Input: part model. Units: mm. Frame: model coordinates. Face numbers are marked on the shaded views. A direction names the side the tool comes from. Coordinates: 2 decimals unless noted, no trailing zeros. Loops run counter-clockwise (first coordinate to the right, second up) from the corner with the lowest first, then second, coordinate; pieces in that order, holes last.
```python
from build123d import *

# Parameters (mm, degrees)
SKETCH1_W           = 24.634
SKETCH1_H           = 13
BOSS_EXTRUDE1_DEPTH = 10
SKETCH4_W           = 70
SKETCH4_H           = 13
BOSS_EXTRUDE4_DEPTH = 15
FILLET2_R           = 5
SKETCH11_R          = 2.68
CUT_EXTRUDE3_DEPTH  = 26
SKETCH12_R          = 4.61
CUT_EXTRUDE4_DEPTH  = 6


with BuildPart() as part:
    # Sketch1 → Boss-Extrude1 (new body)
    with BuildSketch(Plane.XY):
        with Locations((12.317, 6.5)):
            Rectangle(SKETCH1_W, SKETCH1_H)
    extrude(amount=BOSS_EXTRUDE1_DEPTH)

    # Sketch4 → Boss-Extrude4 (add)
    with BuildSketch(Plane.XY.offset(10)):
        with Locations((35, 6.5)):
            Rectangle(SKETCH4_W, SKETCH4_H)
    extrude(amount=BOSS_EXTRUDE4_DEPTH)

    # Fillet2
    fillet2_edges = [part.edges().sort_by_distance(p)[0] for p in [
        (24.634, 6.5, 10),
    ]]
    fillet(fillet2_edges, radius=FILLET2_R)

    # Sketch11 → Cut-Extrude3 (cut, through all)
    with BuildSketch(Plane(origin=(0, 0, 0), x_dir=(-1, 0, 0), z_dir=(0, 0, -1))):
        with Locations((-5.067, 6.5)):
            Circle(SKETCH11_R)
        with Locations((-19.567, 6.5)):
            Circle(SKETCH11_R)
    extrude(amount=-CUT_EXTRUDE3_DEPTH, mode=Mode.SUBTRACT)

    # Sketch12 → Cut-Extrude4 (cut)
    with BuildSketch(Plane.XY.offset(25)):
        with Locations((5.067, 6.5)):
            Circle(SKETCH12_R)
        with Locations((19.567, 6.5)):
            Circle(SKETCH12_R)
    extrude(amount=-CUT_EXTRUDE4_DEPTH, mode=Mode.SUBTRACT)


solid = part.part
```
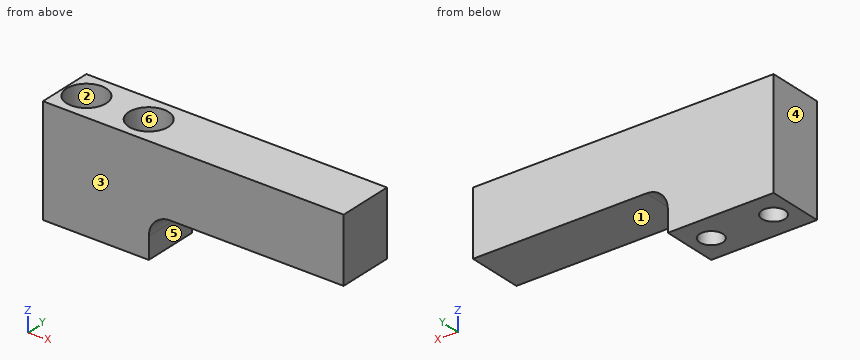
Item 1: Section query A-A (y = 6.5). Output: boundary loops of the cut face in (x, z), then the cut area to 3 significant figures.
Result:
outline: (0, 0) - (2.39, 0) - (2.39, 19) - (0.46, 19) - (0.46, 25) - (0, 25) - close; (7.75, 0) - (16.89, 0) - (16.89, 19) - (14.96, 19) - (14.96, 25) - (9.68, 25) - (9.68, 19) - (7.75, 19) - close; (22.25, 0) - (24.63, 0) - (24.63, 5) arc R5 cw to (29.63, 10) - (70, 10) - (70, 25) - (24.18, 25) - (24.18, 19) - (22.25, 19) - close
area: 987 mm2
Item 2: Mould query, pull axis Y, two halves, no side actions, for the marked faces 1, 2 and 3. Classes: +Y half, -Y half, draft (parallel to the pull), parting line (faces both ways), or undercut.
Result:
face 1: draft
face 2: undercut
face 3: -Y half
Item 3: Section query D-D (z = 21.5). Output: boundary loops of the cut face in (x, y), then the cut area to 3 significant figures.
Result:
outline: (0, 0) - (70, 0) - (70, 13) - (0, 13) - close; hole circle Ø9.22 at (5.07, 6.5); hole circle Ø9.22 at (19.57, 6.5)
area: 776 mm2
Item 4: Contact query for flat-ended pins moving along their axis: P1, Ø7.5, axis at x = 19, y = 6, coming from the +Z side; P2, Ø1.5, axis at x = 63, y = 9, coming from the -Z side; P3, Ø4, axis at y = 3.5, z = 1.5, coming from the +X side. Output: stop coordinate, or through.
Result:
P1: stops at z = 19
P2: stops at z = 10
P3: stops at x = 24.63
Item 5: Reachability of the marked faces 4, 5 and 6 from +Z, -Z, +X, -X, +Y, -Y: full face, straight path, thin tool, end or side. Return the list, or none.
Result:
face 4: +Z, -Z, -X, +Y, -Y
face 5: -Z, +X, +Y, -Y
face 6: +Z
Item 6: Section query B-B (z = 3.5). Output: boundary loops of the cut face in (x, y), then the cut area to 3 significant figures.
Result:
outline: (0, 0) - (24.63, 0) - (24.63, 13) - (0, 13) - close; hole circle Ø5.36 at (5.07, 6.5); hole circle Ø5.36 at (19.57, 6.5)
area: 275 mm2
Item 7: Section query C-C (x = 8.5). Output: boundary loops of the cut face in (y, z), then the cut area to 3 significant figures.
Result:
outline: (0, 0) - (13, 0) - (13, 25) - (9.58, 25) - (9.58, 19) - (3.42, 19) - (3.42, 25) - (0, 25) - close
area: 288 mm2
Item 8: Line query: L1, parallel to X at y = 7, z = 12.5; L2, parallel to X at y = 8.75, z = 13.25; L3, parallel to Y at x = 19.5, z = 21. Output: solid intervals per line, ascending.
Result:
L1: x = 0 to 2.43, 7.7 to 16.93, 22.2 to 70
L2: x = 0 to 3.61, 6.52 to 18.11, 21.02 to 70
L3: y = 0 to 1.89, 11.11 to 13
